Part model, mm, in its own coordinate system. Face numbers are marked on the shaded views. A direction names the side the tool comes from. Round coordinates to 2 decimals unless told otherwise and drop trailing zeros. Write each loop counter-clockwise with the first axis right and the second up, starting at its lowest first coordinate (ties: lowest second). Pieces come first, ordered by that corner, then holes. Notation, with made-up numbers: M 16,31.5 L 43,31.5 A16 cw 43,45.5 Z; hole C 9,84.5 d2. An arc over 180 degrees is marked long. Use a Markdown table: item, result. Add a question column.
1) Slice it at D-D on z = -93. Write the cut outline in (x, y), plus the area to 3 significant figures.
2) Two-plate mould, pull along Z, no slides. Class the marked faces 3, 4 and 5: released by +Z, released by -Z, zero draft, split by the parting line, or undercut.
3) Drop flat-ended pins along their axis: P1, Ø13, axis at y = 0, z = -38, coming from the -X side; P2, Ø12, axis at x = 17.5, z = -136, coming from the -Y side; P3, Ø3, axis at y = 5.5, z = -95, coming from the +X side; P4, Ø2.5, axis at y = -7, z = 0, coming from the +X side. Give the stop position or say it passes through.
4) Slice it at C-C on x = 15.5. Write the cut outline in (y, z).
5) Wall check: probe 1 along Y at (x, z) = (2.5, 0); probe 2 along Y at (x, z) = (14, -150); probe 3 along Y at (x, z) = (8, -72). Give the ranges that are in metal, low to high.
6) Which spindle directions (+Z, -Z, +X, -X, +Y, -Y) get a long thin tool onto all of the face, cutting with end or side? Do the marked faces 1 and 2. Say none if no direction does.
7) Slice it at A-A on x = -1. Write the cut outline in (y, z).
```python
from build123d import *

# Parameters (mm, degrees)
EXTRUDE_1_DEPTH     = 10
SKETCH_2_R          = 10
CUT_EXTRUDE_1_DEPTH = 2
CUT_EXTRUDE_START   = -2
SKETCH_4_R          = 10
CUT_EXTRUDE_2_DEPTH = 2
SKETCH_5_R          = 1.5
SKETCH_5_R_2        = 2.5
CUT_EXTRUDE_3_DEPTH = 158.572205671
SKETCH_7_R          = 6
EXTRUDE_3_DEPTH     = 30
SKETCH_8_R          = 3
CUT_EXTRUDE_4_DEPTH = 168.645459229
CHAMFER_1_SIZE      = 1.5
CUT_EXTRUDE_5_DEPTH = 5
RIB_1_REACH         = 161.389
SKETCH_10_WALL_W    = 454.069017414
SKETCH_10_WALL_H    = 3


with BuildPart() as part:
    # 草图1 → 凸台-拉伸1 (new, symmetric)
    with BuildSketch(Plane(origin=(0, 0, 0), x_dir=(0, 0, -1), z_dir=(1, 0, 0))):
        with BuildLine():
            Line((13, 0), (-13, 0))
            ThreePointArc((-13, 0), (-9.192388155, -9.192388155), (0, -13))
            Line((0, -13), (1.210696705, -12.94350082))
            ThreePointArc((1.210696705, -12.94350082), (9.610906751, -8.753883219), (13, 0))
        make_face()
        with BuildLine():
            ThreePointArc((0.607234259, 12.9858102), (-8.975131047, 9.404627727), (-13, 0))
            Line((-13, 0), (13, 0))
            ThreePointArc((13, 0), (9.404627727, 8.975131047), (0.607234259, 12.9858102))
        make_face()
        with BuildLine():
            ThreePointArc((0.607234259, 12.9858102), (9.404627727, 8.975131047), (13, 0))
            Line((13, 0), (144, 0))
            ThreePointArc((144, 0), (145.757359313, 4.242640687), (150, 6))
            Line((150, 6), (0.607234259, 12.9858102))
        make_face()
        with BuildLine():
            Line((144, 0), (13, 0))
            ThreePointArc((13, 0), (9.610906751, -8.753883219), (1.210696705, -12.94350082))
            Line((1.210696705, -12.94350082), (150, -6))
            ThreePointArc((150, -6), (145.757359313, -4.242640687), (144, 0))
        make_face()
        with BuildLine():
            ThreePointArc((150, 6), (145.757359313, 4.242640687), (144, 0))
            Line((144, 0), (156, 0))
            ThreePointArc((156, 0), (154.242640687, 4.242640687), (150, 6))
        make_face()
        with BuildLine():
            Line((156, 0), (144, 0))
            ThreePointArc((144, 0), (145.757359313, -4.242640687), (150, -6))
            ThreePointArc((150, -6), (154.242640687, -4.242640687), (156, 0))
        make_face()
        with BuildLine():
            ThreePointArc((150, 6), (145.757359313, 4.242640687), (144, 0))
            Line((144, 0), (156, 0))
            ThreePointArc((156, 0), (154.242640687, 4.242640687), (150, 6))
        make_face()
        with BuildLine():
            Line((156, 0), (144, 0))
            ThreePointArc((144, 0), (145.757359313, -4.242640687), (150, -6))
            ThreePointArc((150, -6), (154.242640687, -4.242640687), (156, 0))
        make_face()
    extrude(amount=EXTRUDE_1_DEPTH, both=True)

    # 草图2 → 切除-拉伸1 (cut)
    with BuildSketch(Plane.ZY.offset(10)):
        Circle(SKETCH_2_R)
    extrude(amount=-CUT_EXTRUDE_1_DEPTH, mode=Mode.SUBTRACT)

    # 草图4 → 切除-拉伸2 (cut)
    with BuildSketch(Plane(origin=(10, 0, 0), x_dir=(0, 0, -1), z_dir=(1, 0, 0)).offset(CUT_EXTRUDE_START)):
        with Locations(Location((0, 0, 0), (0, 0, 180))):
            Circle(SKETCH_4_R)
    extrude(amount=CUT_EXTRUDE_2_DEPTH, mode=Mode.SUBTRACT)

    # 草图5 → 切除-拉伸3 (cut, through all)
    with BuildSketch(Plane(origin=(8, 0, 0), x_dir=(0, 0, -1), z_dir=(1, 0, 0))):
        with Locations((7, 0)):
            Circle(SKETCH_5_R)
        with Locations((0, 7)):
            Circle(SKETCH_5_R)
        with Locations((-7, 0)):
            Circle(SKETCH_5_R)
        with Locations((0, -7)):
            Circle(SKETCH_5_R)
        Circle(SKETCH_5_R_2)
    extrude(amount=-CUT_EXTRUDE_3_DEPTH, mode=Mode.SUBTRACT)

    # 草图7 → 凸台-拉伸3 (add, symmetric)
    with BuildSketch(Plane(origin=(0, 0, 0), x_dir=(0, 0, -1), z_dir=(1, 0, 0))):
        with Locations((150, 0)):
            Circle(SKETCH_7_R)
    extrude(amount=EXTRUDE_3_DEPTH, both=True)

    # 草图8 → 切除-拉伸4 (cut, through all)
    with BuildSketch(Plane(origin=(30, 0, 0), x_dir=(0, 0, -1), z_dir=(1, 0, 0))):
        with Locations((150, 0)):
            Circle(SKETCH_8_R)
    extrude(amount=-CUT_EXTRUDE_4_DEPTH, mode=Mode.SUBTRACT)

    # 倒角1
    chamfer_1_edges = [part.edges().sort_by_distance(p)[0] for p in [
        (-30, 0, -144),
        (30, 0, -144),
    ]]
    chamfer(chamfer_1_edges, length=CHAMFER_1_SIZE)

    # 草图9 → 切除-拉伸5 (cut)
    with BuildSketch(Plane.ZY.offset(10)):
        with BuildLine():
            Line((-145.332480771, -5.216729267), (-1.140319123, -11.945696811))
            ThreePointArc((-1.140319123, -11.945696811), (-11.996480106, 0.290628762), (-0.560523931, 11.986901723))
            Line((-0.560523931, 11.986901723), (-145.332945614, 5.217145135))
            ThreePointArc((-145.332945614, 5.217145135), (-143.000000007, 0.000311859), (-145.332480771, -5.216729267))
        make_face()
    cut_extrude_5 = extrude(amount=-CUT_EXTRUDE_5_DEPTH, mode=Mode.SUBTRACT)

    # 镜向1: 切除-拉伸5 across plane
    add(cut_extrude_5.mirror(Plane(origin=(0, 0, 0), x_dir=(0, 0, 1), z_dir=(1, 0, 0))), mode=Mode.SUBTRACT)

    # 草图10 wall → 筋1 (add, up to next)
    with BuildSketch(Plane(origin=(-19.25, 0, -78), x_dir=(0.138795007241, 0, 0.990321132747), z_dir=(0.990321132747, 0, -0.138795007241)), mode=Mode.PRIVATE) as rib_1_sk1:
        Rectangle(SKETCH_10_WALL_W, SKETCH_10_WALL_H)
    rib_1_tool1 = extrude(rib_1_sk1.sketch, amount=RIB_1_REACH, mode=Mode.PRIVATE) - part.part
    rib_1 = rib_1_tool1.solids().sort_by_distance((-19.25, 0, -78))[0]
    add(rib_1)

    # 镜向2: 筋1 across plane
    add(rib_1.mirror(Plane(origin=(0, 0, 0), x_dir=(0, 0, 1), z_dir=(1, 0, 0))))


solid = part.part
```
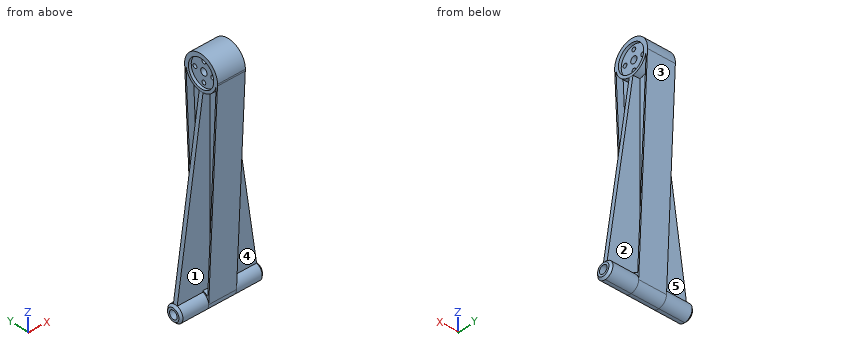
Entries:
| question | item | result |
|---|---|---|
| 1 | outline | M -21.35,-1.5 L -5,-1.5 L -5,-7.66 L -10,-7.66 L -10,-8.66 L 10,-8.66 L 10,-7.66 L 5,-7.66 L 5,-1.5 L 21.35,-1.5 L 21.35,1.5 L 5,1.5 L 5,7.66 L 10,7.66 L 10,8.67 L -10,8.67 L -10,7.66 L -5,7.66 L -5,1.5 L -21.35,1.5 Z |
| 1 | area | 291 mm^2 |
| 2 | face 3 | released by -Z |
| 2 | face 4 | undercut |
| 2 | face 5 | undercut |
| 3 | P1 | stops at x = -14.55 |
| 3 | P2 | stops at y = -1.5 |
| 3 | P3 | stops at x = 5 |
| 3 | P4 | passes through |
| 4 | outline | M -1.5,-144.19 A6 ccw long 1.5,-144.19 L 1.5,-51.24 L -1.5,-51.24 Z; hole C 0,-150 d6 |
| 5 | probe 1 | y = -13 to -8.5, -5.5 to -2.5, 2.5 to 5.5, 8.5 to 13 |
| 5 | probe 2 | y = -6 to -3, 3 to 6 |
| 5 | probe 3 | y = -9.64 to -8.64, -1.5 to 1.5, 8.65 to 9.65 |
| 6 | face 1 | -X |
| 6 | face 2 | +X |
| 7 | outline | M -13,0 L -6,-150 A6 ccw 6,-150 L 12.99,-0.61 A13 ccw long Z; hole C -7,0 d3; hole C 0,-150 d6; hole C 0,0 d5; hole C 0,-7 d3; hole C 0,7 d3; hole C 7,0 d3 |
